Can you work these out from the model? Positions are in its coordinate system, mm. Give positions to 0.01 mm unless a question says otherwise; leave off trailing zeros. Write each loop counter-clockwise with the first axis right and the second up, starting at its lowest first coordinate (ties: lowest second). Pieces come first, ordered by that corner, then holes.
from build123d import *

# Parameters (mm, degrees)
SKETCH_2_W          = 46
SKETCH_2_H          = 46
SKETCH_2_R          = 18
EXTRUDE_1_DEPTH     = 5
FILLET_1_R          = 5.5
SKETCH_3_R          = 1.6
CUT_EXTRUDE_1_DEPTH = 33.908965344
SKETCH_4_R          = 55
SKETCH_4_R_2        = 1.6
SKETCH_4_R_3        = 18
EXTRUDE_2_DEPTH     = 5


with BuildPart() as part:
    # 草图2 → 凸台-拉伸1 (new body)
    with BuildSketch(Plane(origin=(0, 0, 0), x_dir=(1, 0, 0), z_dir=(0, 1, 0))):
        Rectangle(SKETCH_2_W, SKETCH_2_H)
        with Locations(Location((0, 0, 0), (0, 0, 270))):
            Circle(SKETCH_2_R, mode=Mode.SUBTRACT)
    extrude(amount=EXTRUDE_1_DEPTH)

    # 圆角1
    fillet_1_edges = [part.edges().sort_by_distance(p)[0] for p in [
        (23, 2.5, 23),
        (-23, 2.5, 23),
        (-23, 2.5, -23),
        (23, 2.5, -23),
    ]]
    fillet(fillet_1_edges, radius=FILLET_1_R)

    # 草图3 → 切除-拉伸1 (cut, through all)
    with BuildSketch(Plane(origin=(0, 5, 0), x_dir=(1, 0, 0), z_dir=(0, 1, 0))):
        with Locations(Location((-15.5, 15.5, 0), (0, 0, 270))):
            Circle(SKETCH_3_R)
        with Locations(Location((15.5, 15.5, 0), (0, 0, 270))):
            Circle(SKETCH_3_R)
        with Locations(Location((-15.5, -15.5, 0), (0, 0, 270))):
            Circle(SKETCH_3_R)
        with Locations(Location((15.5, -15.5, 0), (0, 0, 270))):
            Circle(SKETCH_3_R)
    extrude(amount=-CUT_EXTRUDE_1_DEPTH, mode=Mode.SUBTRACT)

    # 草图4 → 凸台-拉伸2 (add)
    # profile 1 of 2: a face of its own
    with BuildSketch(Plane(origin=(0, 5, 0), x_dir=(1, 0, 0), z_dir=(0, 1, 0))):
        with Locations(Location((0, 0, 0), (0, 0, 270))):
            Circle(SKETCH_4_R)
        with Locations(Location((-49.1, 0, 0), (0, 0, 270))):
            Circle(SKETCH_4_R_2, mode=Mode.SUBTRACT)
        with Locations(Location((0, -49.1, 0), (0, 0, 270))):
            Circle(SKETCH_4_R_2, mode=Mode.SUBTRACT)
        with Locations(Location((49.1, 0, 0), (0, 0, 270))):
            Circle(SKETCH_4_R_2, mode=Mode.SUBTRACT)
        with Locations(Location((0, 49.1, 0), (0, 0, 270))):
            Circle(SKETCH_4_R_2, mode=Mode.SUBTRACT)
        with BuildLine():
            Line((-17.5, -23), (17.5, -23))
            ThreePointArc((17.5, -23), (21.389087297, -21.389087297), (23, -17.5))
            Line((23, -17.5), (23, 17.5))
            ThreePointArc((23, 17.5), (21.389087297, 21.389087297), (17.5, 23))
            Line((17.5, 23), (-17.5, 23))
            ThreePointArc((-17.5, 23), (-21.389087297, 21.389087297), (-23, 17.5))
            Line((-23, 17.5), (-23, -17.5))
            ThreePointArc((-23, -17.5), (-21.389087297, -21.389087297), (-17.5, -23))
        make_face(mode=Mode.SUBTRACT)
    # profile 2 of 2: a face of its own
    with BuildSketch(Plane(origin=(0, 5, 0), x_dir=(1, 0, 0), z_dir=(0, 1, 0))):
        with BuildLine():
            ThreePointArc((-23, -17.5), (-21.389087297, -21.389087297), (-17.5, -23))
            Line((-17.5, -23), (17.5, -23))
            ThreePointArc((17.5, -23), (21.389087297, -21.389087297), (23, -17.5))
            Line((23, -17.5), (23, 17.5))
            ThreePointArc((23, 17.5), (21.389087297, 21.389087297), (17.5, 23))
            Line((17.5, 23), (-17.5, 23))
            ThreePointArc((-17.5, 23), (-21.389087297, 21.389087297), (-23, 17.5))
            Line((-23, 17.5), (-23, -17.5))
        make_face()
        with Locations(Location((15.5, 15.5, 0), (0, 0, 270))):
            Circle(SKETCH_4_R_2, mode=Mode.SUBTRACT)
        with Locations(Location((-15.5, -15.5, 0), (0, 0, 270))):
            Circle(SKETCH_4_R_2, mode=Mode.SUBTRACT)
        with Locations(Location((0, 0, 0), (0, 0, 270))):
            Circle(SKETCH_4_R_3, mode=Mode.SUBTRACT)
        with Locations(Location((-15.5, 15.5, 0), (0, 0, 270))):
            Circle(SKETCH_4_R_2, mode=Mode.SUBTRACT)
        with Locations(Location((15.5, -15.5, 0), (0, 0, 270))):
            Circle(SKETCH_4_R_2, mode=Mode.SUBTRACT)
    extrude(amount=-EXTRUDE_2_DEPTH)


solid = part.part
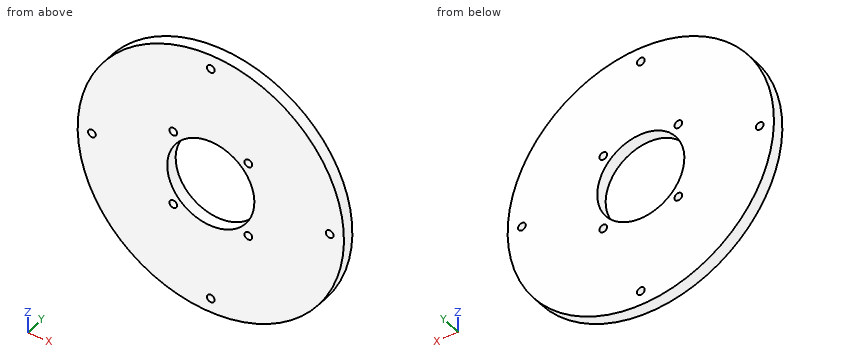
(1) Imagine slicing it at C-C, the plane y = 0.85. Give the number of separate pieces and of enclosed holes in the cut face, plus the area to 3 significant figures.
Returned:
separate pieces: 1
enclosed holes: 9
area: 8,420 mm2
(2) Imagine slicing it at A-A, the plane x = 0. Write out the boundary of the cut face in (y, z), plus the area to 3 significant figures.
Returned:
outline: (0, -55) - (5, -55) - (5, -50.7) - (0, -50.7) - close; (0, -47.5) - (5, -47.5) - (5, -18) - (0, -18) - close; (0, 18) - (5, 18) - (5, 47.5) - (0, 47.5) - close; (0, 50.7) - (5, 50.7) - (5, 55) - (0, 55) - close
area: 338 mm2
(3) Imagine slicing it at D-D, the plane x = 49.1. Write out the boundary of the cut face in (y, z).
Returned:
outline: (0, -24.78) - (5, -24.78) - (5, -1.6) - (0, -1.6) - close; (0, 1.6) - (5, 1.6) - (5, 24.78) - (0, 24.78) - close
(4) If I drill on L1, parallel to X at y = 1.55, z = 0; L2, parallel to X at y = 1.25, z = 15.5; L3, parallel to X at y = 3.25, z = -4, over which ranges is the centre line in solid material (lowest first)?
Returned:
L1: x = -55 to -50.7, -47.5 to -18, 18 to 47.5, 50.7 to 55
L2: x = -52.77 to -17.1, -13.9 to -9.15, 9.15 to 13.9, 17.1 to 52.77
L3: x = -54.85 to -17.55, 17.55 to 54.85
(5) Imagine slicing it at B-B, the plane z = -49.1. Write out the boundary of the cut face in (x, y), plus the area to 3 significant figures.
Returned:
outline: (-24.78, 0) - (-1.6, 0) - (-1.6, 5) - (-24.78, 5) - close; (1.6, 0) - (24.78, 0) - (24.78, 5) - (1.6, 5) - close
area: 232 mm2
(6) Will these pins go through, and if not, where does the flat tip stop? P1, Ø4, axis at x = -15.5, z = 15.5, coming from the +Y side; P2, Ø1.9, axis at x = 15.5, z = -15.5, coming from the +Y side; P3, Ø1.5, axis at x = -22.5, y = 1, coming from the +Z side; P4, Ø1, axis at x = -2, y = 0.5, coming from the -Z side.
Returned:
P1: stops at y = 5
P2: passes through
P3: stops at z = 50.52
P4: stops at z = -54.98
